from build123d import *

# Parameters (mm, degrees)
F0_R     = 1.5
F0_R_2   = 1.45
F0_R_3   = 4.75
F1_DEPTH = 3
F2_R     = 5


with BuildPart() as f1:
    # F0 (on Top) → F1 (new body)
    with BuildSketch(Plane.XY):
        Polygon((67.5, 27.96), (27.96, 67.5), (-27.96, 67.5), (-67.5, 27.96), (-67.5, -27.96), (-27.96, -67.5), (27.96, -67.5), (67.5, -27.96), align=None)
        with Locations((-9.5, -54.5)):
            Circle(F0_R, mode=Mode.SUBTRACT)
        with Locations((-54.5, -9.5)):
            Circle(F0_R, mode=Mode.SUBTRACT)
        with Locations((-9.5, -18.5)):
            Circle(F0_R_2, mode=Mode.SUBTRACT)
        with Locations((-18.5, -9.5)):
            Circle(F0_R_2, mode=Mode.SUBTRACT)
        with Locations((9.5, -54.5)):
            Circle(F0_R, mode=Mode.SUBTRACT)
        with Locations((0, -21.215)):
            Circle(F0_R_2, mode=Mode.SUBTRACT)
        with Locations((9.5, -18.5)):
            Circle(F0_R_2, mode=Mode.SUBTRACT)
        with Locations((18.5, -9.5)):
            Circle(F0_R_2, mode=Mode.SUBTRACT)
        with Locations((54.5, -9.5)):
            Circle(F0_R, mode=Mode.SUBTRACT)
        with Locations((-54.5, 9.5)):
            Circle(F0_R, mode=Mode.SUBTRACT)
        with Locations((-21.215, 0)):
            Circle(F0_R_2, mode=Mode.SUBTRACT)
        with Locations((-18.5, 9.5)):
            Circle(F0_R_2, mode=Mode.SUBTRACT)
        with Locations((-9.5, 18.5)):
            Circle(F0_R_2, mode=Mode.SUBTRACT)
        with Locations((-9.5, 54.5)):
            Circle(F0_R, mode=Mode.SUBTRACT)
        Circle(F0_R_3, mode=Mode.SUBTRACT)
        with Locations((21.215, 0)):
            Circle(F0_R_2, mode=Mode.SUBTRACT)
        with Locations((18.5, 9.5)):
            Circle(F0_R_2, mode=Mode.SUBTRACT)
        with Locations((0, 21.215)):
            Circle(F0_R_2, mode=Mode.SUBTRACT)
        with Locations((9.5, 18.5)):
            Circle(F0_R_2, mode=Mode.SUBTRACT)
        with Locations((54.5, 9.5)):
            Circle(F0_R, mode=Mode.SUBTRACT)
        with Locations((9.5, 54.5)):
            Circle(F0_R, mode=Mode.SUBTRACT)
    extrude(amount=F1_DEPTH)

    # F2
    f2_edges = [f1.edges().sort_by_distance(p)[0] for p in [
        (-27.96, 67.5, 1.5),
        (-67.5, 27.96, 1.5),
        (-67.5, -27.96, 1.5),
        (-27.96, -67.5, 1.5),
        (27.96, -67.5, 1.5),
        (67.5, -27.96, 1.5),
        (67.5, 27.96, 1.5),
        (27.96, 67.5, 1.5),
    ]]
    fillet(f2_edges, radius=F2_R)


solid = f1.part
CAD build for the part. Positions are in the model's coordinates, mm. Round coordinates to 2 decimals unless told otherwise and drop trailing zeros. Order: outer loops, then holes, each group sorted by start corner. A loop starts at its lowest first (then second) coordinate and runs counter-clockwise, first axis right, second up. Notation, with made-up numbers: (64.5, -17) -> (107.5, -17) arc R14 ccw to (107.5, -3) -> close; hole circle Ø1 at (-24.75, 65). An arc over 180 degrees is marked (long way). Write item = value, one per line. Start each with the question number.
(1) Probe line 1 (Y direction, x = -9.5, z = 1.6); line 2 (Y direction, x = -21, z = 1.6); line 3 (X direction, y = -0.5, z = 1.6). List the from-to ranges inside material, lowest first. Write a range as [from, to].
(2) Cut at B-B, the plane y = 34. List the corners of the cut face in (x, z).
(3) Cut at A-A, the plane x = 38. List the corners of the cut face in (y, z), then the cut area to 3 significant figures.
(4) Pull direction Y, two halves, no side cores. Call faces 1 (the flat face through (47.47, -47.99, 1.48)), 2 (the flat face through (-1, 16, 3)), 3 (the cylindrical face through (-17.161, -10.055, 1.479)): released by +Y, released by -Y, zero draft, split by the parting line, or undercut.
(5) Cut at C-C, the plane z = 2.35. State how many separate pieces and enclosed holes the cut face has, then the cut area to 3 significant figures.
Model answer:
q1.line_1 = [-67.5, -56], [-53, -19.95], [-17.05, 17.05], [19.95, 53], [56, 67.5]
q1.line_2 = [-67.5, -1.43], [1.43, 67.5]
q1.line_3 = [-67.5, -22.58], [-19.85, -4.72], [4.72, 19.85], [22.58, 67.5]
q2.outline = (-61.46, 0) -> (61.46, 0) -> (61.46, 3) -> (-61.46, 3) -> close
q3.outline = (-57.46, 0) -> (57.46, 0) -> (57.46, 3) -> (-57.46, 3) -> close
q3.area = 345 mm2
q4.face_1 = released by -Y
q4.face_2 = zero draft
q4.face_3 = undercut
q5.separate_pieces = 1
q5.enclosed_holes = 21
q5.area = 14,900 mm2
